Answer from the drawing. Dimensions are ordinates in mm from the lowest x, y and z of the part. Round coordinates to 2 decimals unless told otherwise and drop trailing zeros. Write each loop counter-clockwise with the first axis right and the second up, starting at its lowest first coordinate (ties: lowest second). Pieces come first, ordered by that corner, then holes. Notation, with made-up numbers: (58, 38) - (82, 38) arc R22 cw to (82, 64) - close; hole circle Ø9 at (88, 23.5). An arc over 180 degrees is marked (long way). One line per item, written item: value. Start each with the question number.
(1) Find the intervals of material crossed by L1, parallel to X at y = 2, z = 0.2; L2, parallel to Y at x = 29.4, z = 0.1, in increasing order.
(2) A flat-ended cylindrical pin translates along its axis: pin 1 Ø1.4 at (x, y) = (29.4, 2) entering from -Z. Find the tip coordinate at first contact, or state that the pin passes through.
(3) A cutting plane is placed at A-A, the plane x = 29.4. Determine the outline of the cut face in (y, z).
(4) A cutting plane is placed at B-B, the plane z = 0.6. Determine the outline of the cut face in (x, y).
(5) A cutting plane is placed at C-C, the plane y = 25.4. Determine the outline of the cut face in (x, z).
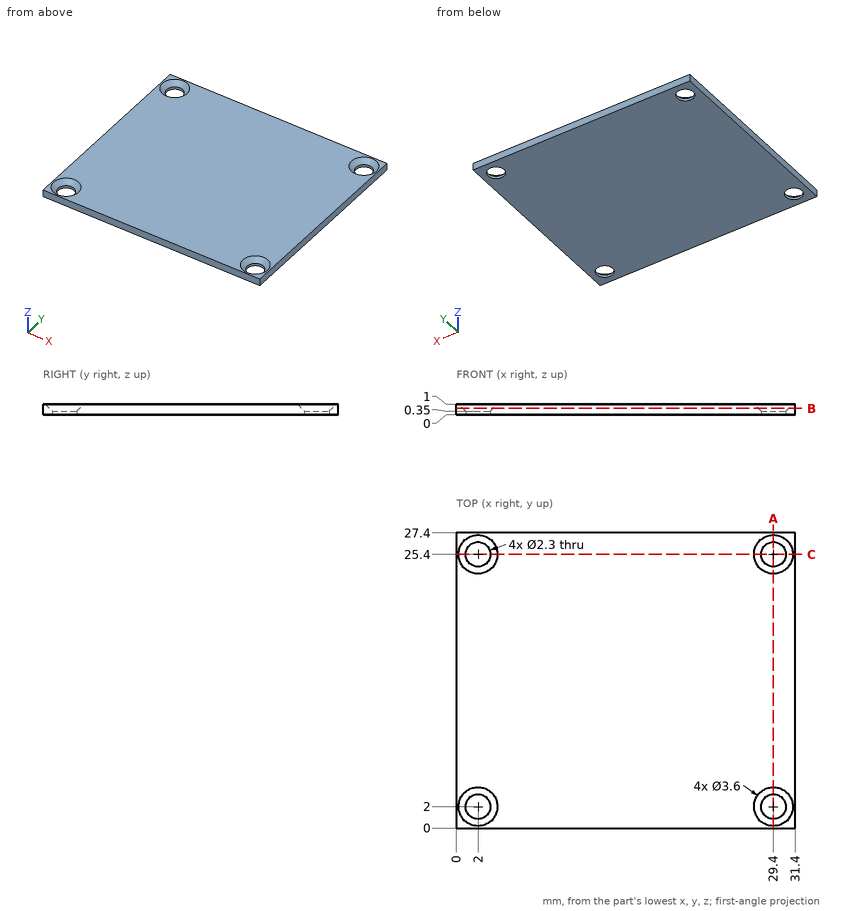
Here are the results:
1. L1: 0 to 0.85, 3.15 to 28.25, 30.55 to 31.4
1. L2: 0 to 0.85, 3.15 to 24.25, 26.55 to 27.4
2. pin 1: through
3. outline: (0, 0) - (0.85, 0) - (0.85, 0.35) - (0.2, 1) - (0, 1) - close; (3.15, 0) - (24.25, 0) - (24.25, 0.35) - (23.6, 1) - (3.8, 1) - (3.15, 0.35) - close; (26.55, 0) - (27.4, 0) - (27.4, 1) - (27.2, 1) - (26.55, 0.35) - close
4. outline: (0, 0) - (31.4, 0) - (31.4, 27.4) - (0, 27.4) - close; hole circle Ø2.8 at (2, 2); hole circle Ø2.8 at (2, 25.4); hole circle Ø2.8 at (29.4, 2); hole circle Ø2.8 at (29.4, 25.4)
5. outline: (0, 0) - (0.85, 0) - (0.85, 0.35) - (0.2, 1) - (0, 1) - close; (3.15, 0) - (28.25, 0) - (28.25, 0.35) - (27.6, 1) - (3.8, 1) - (3.15, 0.35) - close; (30.55, 0) - (31.4, 0) - (31.4, 1) - (31.2, 1) - (30.55, 0.35) - close
